The listing builds one solid part. Answer for the finished solid, in the listing's coordinates (mm). A direction names the side the tool comes from. Coordinates: 2 decimals unless noted, no trailing zeros. Order: outer loops, then holes, each group sorted by start corner. A loop starts at its lowest first (then second) coordinate and runs counter-clockwise, first axis right, second up. Notation, with made-up numbers: (45.25, 29.5) - (80.25, 29.5) arc R16 cw to (80.25, 55.5) - close; hole circle Ø2 at (12.25, -20.5). An arc over 180 degrees is marked (long way). Use a Markdown table: item, result. Add a question column.
Item 1: The part is cut by section B-B, the plane z = -10.5. Give the vertices of the cut face in (x, y).
Item 2: The mould has two halves that part along X. Classify faces 1 (the flat face through (0, -38.935, 12)), 2 (the flat face through (0, -38.935, -24)), 3 (the cylindrical face through (-2.98, -40.66, -22.69)): released by +X, released by -X, zero draft, split by the parting line, or undercut.
Item 3: Flat-ended cylindrical pins translate along their axes: P1, Ø1.5, axis at x = 25, y = -14, coming from the +Z side; P2, Ø1.5, axis at x = -24.5, z = -0.5, coming from the -Y side; P3, Ø1, axis at y = -24.5, z = 34, coming from the -X side. Find the tip coordinate at first contact, or state that the pin passes through.
Item 4: The part is cut by section C-C, the plane z = -24.5. Give the vertices of the cut face in (x, y), then the cut area to 3 significant figures.
Item 5: For faces 4 (the flat face through (0, -42.435, 0)), 5 (the flat face through (0, -38.935, 24)), 6 (the conical face through (2, 45, 5)), determine the directions among +Z, -Z, +X, -X, +Y, -Y from which every point of the face is accessible in a straight line to the end or side of a thin tool.
Item 6: The part is cut by section A-A, the plane z = 0. Give the vertices of the cut face in (x, y).
Item 7: Find the intervals of material crossed by line 1 along Z through (x, y) = (-12, 8.5); line 2 along Y through (x, z) = (16, -35.5); line 3 along X through (y, z) = (15, 39.5), in increasing order.
Solid Edge part; units mm, degrees
sketch "Sketch1" plane through (0, 0, 0) normal (0, -1, 0) x (1, 0, 0)
  line L0 (44.7214, 5) -> (49.7494, 5)
  line L1 (0, 45) -> (0, 50)
  arc A0 (0, 50) -> (49.7494, 5) centre (0, 0) cw
  arc A1 (0, 45) -> (44.7214, 5) centre (0, 0) cw
revolve "RevolvedProtrusion1" add sketch "Sketch1" angle 360 about axis through (0, 0, 45) along (0, 0, 1)
sketch "Sketch2" plane through (0, 0, 0) normal (0, -1, 0) x (1, 0, 0)
  line L0 (0, 5.2892) -> (44.6881, 5.2892)
  arc A0 (44.6881, 5.2892) -> (44.7214, -5) centre (0, 0) cw
  line L1 (0, -5) -> (44.7214, -5)
  line L2 (0, -5) -> (0, 5.2892)
revolve "RevolvedProtrusion2" add sketch "Sketch2" angle 360 about axis through (0, 0, -5) along (0, 0, 1)
sketch "Sketch3" plane through (0, 0, 0) normal (0, -1, 0) x (1, 0, 0)
  line L0 (0, -5) -> (0, -50)
  line L1 (49.7494, -5) -> (0, -5)
  arc A0 (49.7494, -5) -> (0, -50) centre (0, 0) cw
revolve "RevolvedProtrusion3" add sketch "Sketch3" angle 360 about axis through (0, 0, -5) along (0, 0, -1)
extrude "Cutout1" [suppressed]
sketch "Sketch4" plane through (0, -38.9353, 0) normal (0, -1, 0) x (1, 0, 0)
  circle A0 centre (0, 0.1446) radius 45.8242
extrude "Cutout2" cut sketch "Sketch4" along normal blind 20
sketch "Sketch5" plane through (0, -38.9353, 0) normal (0, -1, 0) x (1, 0, 0)
  circle A0 centre (0, 0) radius 22.8836
extrude "ExtrudedProtrusion_1" add sketch "Sketch5" along normal blind 3.5
Solution:
| question | item | result |
|---|---|---|
| 1 | outline | (-29.56, -38.94) - (-20.33, -38.94) - (-20.33, -42.44) - (20.33, -42.44) - (20.33, -38.94) - (29.56, -38.94) arc R48.89 ccw (long way) to start |
| 2 | face 1 | undercut |
| 2 | face 2 | zero draft |
| 2 | face 3 | split by the parting line |
| 3 | P1 | stops at z = 41.49 |
| 3 | P2 | stops at y = -38.22 |
| 3 | P3 | stops at x = -28.03 |
| 4 | outline | (-19.59, -38.94) - (19.59, -38.94) arc R43.59 ccw (long way) to start |
| 4 | area | 5,850 mm2 |
| 5 | face 4 | +Z, -Z, +X, -X, -Y |
| 5 | face 5 | +Z, -Y |
| 5 | face 6 | none |
| 6 | outline | (-22.88, -42.44) - (22.88, -42.44) - (22.88, -38.94) - (22.56, -38.94) arc R45 ccw (long way) to (-22.56, -38.94) - (-22.88, -38.94) - close |
| 7 | line 1 | z = -47.79 to 5.29, 42.53 to 47.79 |
| 7 | line 2 | y = -31.36 to 31.36 |
| 7 | line 3 | x = -26.73 to -15.48, 15.48 to 26.73 |
